The listing builds one solid part. Answer for the finished solid, in the listing's coordinates (mm). Give positions to 0.01 mm unless a question says otherwise; leave off trailing zeros. Write each loop counter-clockwise with the first axis right and the second up, starting at its lowest first coordinate (ties: lowest second). Pieces come first, ordered by that corner, then holes.
```python
from build123d import *

# Parameters (mm, degrees)
BOSS_EXTRUDE1_DEPTH   = 60
F_2_5MM_DOWEL_HOLE1_D = 2.5


with BuildPart() as part:
    # Sketch1 → Boss-Extrude1 (new body)
    with BuildSketch(Plane.XY):
        with BuildLine():
            Line((-1.975, 0), (1.975, 0))
            ThreePointArc((1.975, 0), (3.464517951, 5.200996445), (7.481435424, 8.825))
            Line((7.481435424, 8.825), (7.481435424, 9.825))
            Line((7.481435424, 9.825), (-7.481435424, 9.825))
            Line((-7.481435424, 9.825), (-7.481435424, 8.825))
            ThreePointArc((-7.481435424, 8.825), (-3.464517951, 5.200996445), (-1.975, 0))
        make_face()
    extrude(amount=BOSS_EXTRUDE1_DEPTH)

    # Ø2.5mm Dowel Hole1 (through all)
    with Locations(Plane(origin=(0, 9.825, 45), x_dir=(0, 0, 1), z_dir=(0, 1, 0))):
        with Locations((0, 0), (-30, 0)):
            Hole(F_2_5MM_DOWEL_HOLE1_D / 2)


solid = part.part
```
Item 1: Determine the mould class of faces 1 (the face through (0.05, 4.84, 16.25)), 2 (the face through (0, 6, 0)), 3 (the face through (0, 6, 60)), 4 (the face through (3.424, 5.136, 29.58)) for opening direction Z: pulls with the +Z half, pulls with the -Z half, needs draft (parallel to the pull), parting line crosses it, or undercut.
Conclusion:
face 1: undercut
face 2: pulls with the -Z half
face 3: pulls with the +Z half
face 4: needs draft
Item 2: Consider probe 1 along Z at (x, y) = (-1, 7.25); probe 2 along X at (y, z) = (7, 15); probe 3 along X at (y, z) = (3.5, 44.5). Determine where each line is inside the solid, lowest interval first.
Conclusion:
probe 1: z = 0 to 14.25, 15.75 to 44.25, 45.75 to 60
probe 2: x = -4.91 to -1.25, 1.25 to 4.91
probe 3: x = -2.62 to -1.15, 1.15 to 2.62
Item 3: A cutting plane is placed at B-B, the plane z = 45. Give the vertices of the cut face in (x, y) (3 decimals).
Conclusion:
outline: (-7.481, 8.825) arc R9.825 cw to (-1.975, 0) - (-1.25, 0) - (-1.25, 9.825) - (-7.481, 9.825) - close; (1.25, 0) - (1.975, 0) arc R9.825 cw to (7.481, 8.825) - (7.481, 9.825) - (1.25, 9.825) - close
Item 4: A cutting plane is placed at A-A, the plane x = 0. Give the vertices of the cut face in (y, z) (3 decimals).
Conclusion:
outline: (0, 0) - (9.825, 0) - (9.825, 13.75) - (0, 13.75) - close; (0, 16.25) - (9.825, 16.25) - (9.825, 43.75) - (0, 43.75) - close; (0, 46.25) - (9.825, 46.25) - (9.825, 60) - (0, 60) - close
Item 5: A cutting plane is placed at C-C, the plane y = 6. Give the vertices of the cut face in (x, z).
Conclusion:
outline: (-4.02, 0) - (4.02, 0) - (4.02, 60) - (-4.02, 60) - close; hole circle Ø2.5 at (0, 15); hole circle Ø2.5 at (0, 45)
Item 6: A cutting plane is placed at D-D, the plane x = -6.5. Give the vertices of the cut face in (y, z) (3 decimals).
Conclusion:
outline: (8.273, 0) - (9.825, 0) - (9.825, 60) - (8.273, 60) - close
Item 7: Each of these flat-tipped pins is pushed along its axis until it touches: P1, Ø1.5, axis at y = 4.5, z = 19, coming from the +X side; P2, Ø2, axis at x = 0, z = 45, coming from the +Y side; P3, Ø3, axis at x = 6, z = 8.5, coming from the -Y side. Where does it stop, or does it pass through?
Conclusion:
P1: stops at x = 3.5
P2: passes through
P3: stops at y = 6.58
